Can you work these out from the model? Positions are in its coordinate system, mm. Face numbers are marked on the shaded views. A direction names the side the tool comes from. Round coordinates to 2 decimals unless told otherwise and drop trailing zeros. Order: outer loops, then holes, each group sorted by start corner. A loop starts at its lowest first (then second) coordinate and runs counter-clockwise, first axis right, second up. Notation, with made-up numbers: (42, 59.5) -> (90, 59.5) arc R20 cw to (90, 72.5) -> close; hole circle Ø11 at (-16, 21.25). An arc over 180 degrees is marked (long way). One line per item, written item: value.
```python
from build123d import *

# Parameters (mm, degrees)
CROQUIS1_W              = 28
CROQUIS1_H              = 12
SALIENTE_EXTRUIR1_DEPTH = 3
CROQUIS2_R              = 1
CORTAR_EXTRUIR1_DEPTH   = 3
CROQUIS3_W              = 3
CROQUIS3_H              = 8.392153605
SALIENTE_EXTRUIR2_DEPTH = 8
CROQUIS4_R              = 1
CORTAR_EXTRUIR2_DEPTH   = 3
CORTAR_EXTRUIR3_DEPTH   = 8
SALIENTE_EXTRUIR3_START = -7
CROQUIS8_R              = 2
CROQUIS8_R_2            = 1
SALIENTE_EXTRUIR3_DEPTH = 7
SALIENTE_EXTRUIR4_START = 0.5
CROQUIS11_R             = 1
SALIENTE_EXTRUIR4_DEPTH = 0.5
CROQUIS12_R             = 1
SALIENTE_EXTRUIR5_DEPTH = 0.5


with BuildPart() as part:
    # Croquis1 → Saliente-Extruir1 (new body)
    with BuildSketch(Plane.XY):
        with Locations((-16.412225504, 7.356643357)):
            Rectangle(CROQUIS1_W, CROQUIS1_H)
    extrude(amount=SALIENTE_EXTRUIR1_DEPTH)

    # Croquis2 → Cortar-Extruir1 (cut)
    with BuildSketch(Plane.XY.offset(3)):
        with Locations((-26.412225504, 5.356643357)):
            Circle(CROQUIS2_R)
        with Locations((-6.412225504, 5.356643357)):
            Circle(CROQUIS2_R)
    extrude(amount=-CORTAR_EXTRUIR1_DEPTH, mode=Mode.SUBTRACT)

    # Croquis3 → Saliente-Extruir2 (add)
    with BuildSketch(Plane(origin=(0, 0, 0), x_dir=(-1, 0, 0), z_dir=(0, 0, -1))):
        with Locations((16.412225504, 9.160566555)):
            Rectangle(CROQUIS3_W, CROQUIS3_H)
    extrude(amount=SALIENTE_EXTRUIR2_DEPTH)

    # Croquis4 → Cortar-Extruir2 (cut)
    with BuildSketch(Plane.ZY.offset(17.912225504)):
        with Locations((-4.5, 9.856643357)):
            Circle(CROQUIS4_R)
    extrude(amount=-CORTAR_EXTRUIR2_DEPTH, mode=Mode.SUBTRACT)

    # Croquis6 → Cortar-Extruir3 (cut)
    with BuildSketch(Plane.ZY.offset(17.912225504)):
        with BuildLine():
            Line((-8, 13.356643357), (-4.5, 13.356643357))
            Line((-4.5, 13.356643357), (0, 13.356643357))
            Line((0, 13.356643357), (0, 13.306643357))
            Line((0, 13.306643357), (-4.5, 13.306643357))
            ThreePointArc((-4.5, 13.306643357), (-7.95, 9.856643357), (-4.5, 6.406643357))
            Line((-4.5, 6.406643357), (0, 6.406643357))
            Line((0, 6.406643357), (0, 4.964489752))
            Line((0, 4.964489752), (-8, 4.964489752))
            Line((-8, 4.964489752), (-8, 6.352103478))
            Line((-8, 6.352103478), (-8, 13.356643357))
        make_face()
    extrude(amount=-CORTAR_EXTRUIR3_DEPTH, mode=Mode.SUBTRACT)

    # Croquis8 → Saliente-Extruir3 (add)
    # profile 1 of 2: a face of its own
    with BuildSketch(Plane(origin=(0, 0, 0), x_dir=(-1, 0, 0), z_dir=(0, 0, -1)).offset(SALIENTE_EXTRUIR3_START)):
        with Locations((6.412225504, 5.356643357)):
            Circle(CROQUIS8_R)
        with Locations(Location((6.412225504, 5.356643357, 0), (0, 0, 180))):
            Circle(CROQUIS8_R_2, mode=Mode.SUBTRACT)
    # profile 2 of 2: a face of its own
    with BuildSketch(Plane(origin=(0, 0, 0), x_dir=(-1, 0, 0), z_dir=(0, 0, -1)).offset(SALIENTE_EXTRUIR3_START)):
        with Locations((26.412225504, 5.356643357)):
            Circle(CROQUIS8_R)
        with Locations(Location((26.412225504, 5.356643357, 0), (0, 0, 180))):
            Circle(CROQUIS8_R_2, mode=Mode.SUBTRACT)
    extrude(amount=SALIENTE_EXTRUIR3_DEPTH)

    # Croquis11 → Saliente-Extruir4 (add)
    with BuildSketch(Plane.ZY.offset(17.912225504).offset(SALIENTE_EXTRUIR4_START)):
        with BuildLine():
            Line((-4.5, 6.406643357), (0, 6.406643357))
            Line((0, 6.406643357), (0, 13.306643357))
            Line((0, 13.306643357), (-4.5, 13.306643357))
            ThreePointArc((-4.5, 13.306643357), (-7.95, 9.856643357), (-4.5, 6.406643357))
        make_face()
        with Locations((-4.5, 9.856643357)):
            Circle(CROQUIS11_R, mode=Mode.SUBTRACT)
    extrude(amount=-SALIENTE_EXTRUIR4_DEPTH)

    # Croquis12 → Saliente-Extruir5 (add)
    with BuildSketch(Plane(origin=(-14.912225504, 0, 0), x_dir=(0, 0, -1), z_dir=(1, 0, 0))):
        with BuildLine():
            Line((4.5, 13.306643357), (0, 13.306643357))
            Line((0, 13.306643357), (0, 6.406643357))
            Line((0, 6.406643357), (4.5, 6.406643357))
            ThreePointArc((4.5, 6.406643357), (7.95, 9.856643357), (4.5, 13.306643357))
        make_face()
        with Locations(Location((4.5, 9.856643357, 0), (0, 0, 180))):
            Circle(CROQUIS12_R, mode=Mode.SUBTRACT)
    extrude(amount=SALIENTE_EXTRUIR5_DEPTH)


solid = part.part
```
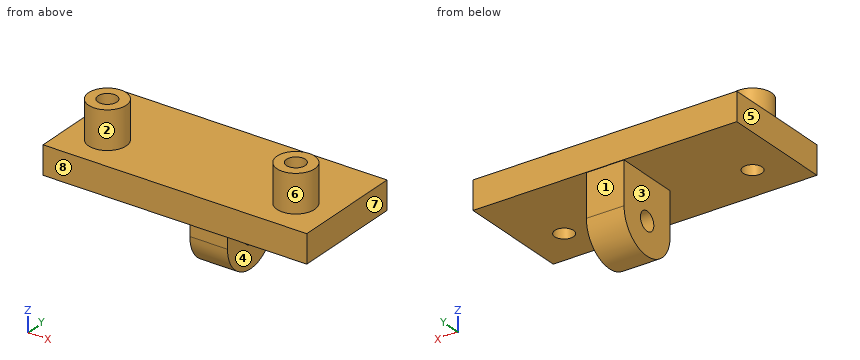
Q1. I want a section at C-C on z = 5.75. List the corners of the cut face in (x, y) for me.
Answers below:
outline: circle Ø4 at (-26.41, 5.36); circle Ø4 at (-6.41, 5.36); hole circle Ø2 at (-26.41, 5.36); hole circle Ø2 at (-6.41, 5.36)
Q2. I want a section at B-B on y = 10.5. List the corners of the cut face in (x, z) for me.
Answers below:
outline: (-30.41, 0) -> (-18.41, 0) -> (-18.41, -3.73) -> (-14.41, -3.73) -> (-14.41, 0) -> (-2.41, 0) -> (-2.41, 3) -> (-30.41, 3) -> close; (-18.41, -7.89) -> (-14.41, -7.89) -> (-14.41, -5.27) -> (-18.41, -5.27) -> close
Q3. On a 3-axis mill with a long thin cutter (end or side, diameter ignored), from which of +Z, -Z, +X, -X, +Y, -Y can I reach the whole of each face in a straight line? I mean the marked faces 1, 2, 3, 4 and 5. Say none if no direction works.
Answers below:
face 1: -Z, +X, -X, +Y
face 2: +Z
face 3: -Z, -X, +Y, -Y
face 4: -Z, +X, +Y, -Y
face 5: +Z, -Z, -X, +Y, -Y
Q4. Please list where these lines run through material, in increasing order: line 1 along Z through (x, y) = (-15, 8); line 2 along Z through (x, y) = (-25.5, 2.75); line 3 along Y through (x, z) = (-16.5, -4.5).
Answers below:
line 1: -7.41 to 3
line 2: 0 to 3
line 3: 6.41 to 8.86, 10.86 to 13.31
Q5. Will these pins go through, and if not, where does the flat tip stop? pin 1 Ø2 at (x, z) = (-16.5, -1.5) entering from +Y; pin 2 Ø3 at (y, z) = (6, -4) entering from +X; pin 3 Ø5.5 at (y, z) = (11, -6) entering from -X; pin 4 Ø1.6 at (x, y) = (-26.41, 5.36) entering from -Z.
Answers below:
pin 1: y = 13.31
pin 2: x = -14.41
pin 3: x = -18.41
pin 4: through
Q6. We'd pull the mould along X, two halves only. Please class the marked faces 6, 7 and 8: released by +X, released by -X, zero draft, split by the parting line, or undercut.
Answers below:
face 6: undercut
face 7: released by +X
face 8: zero draft
Q7. I want a section at D-D on x = -17. List the corners of the cut face in (y, z) for me.
Answers below:
outline: (1.36, 0) -> (6.41, 0) -> (6.41, -4.5) arc R3.45 ccw to (13.31, -4.5) -> (13.31, 0) -> (13.36, 0) -> (13.36, 3) -> (1.36, 3) -> close; hole circle Ø2 at (9.86, -4.5)
Q8. I want a section at A-A on x = -27. List the corners of the cut face in (y, z) for me.
Answers below:
outline: (1.36, 0) -> (4.55, 0) -> (4.55, 7) -> (3.44, 7) -> (3.44, 3) -> (1.36, 3) -> close; (6.17, 0) -> (13.36, 0) -> (13.36, 3) -> (7.27, 3) -> (7.27, 7) -> (6.17, 7) -> close
